Can you work these out from the model? Positions are in its coordinate system, mm. Round coordinates to 2 decimals unless told otherwise and drop trailing zeros. Order: outer loops, then holes, each group sorted by start corner. A loop starts at its lowest first (then second) coordinate and runs counter-clockwise, first axis right, second up. Notation, with made-up numbers: M 20,10.5 L 66,10.5 A16 ccw 66,39.5 Z; hole C -29,63 d11. An arc over 180 degrees is marked long. One line per question, with ' | ' between items.
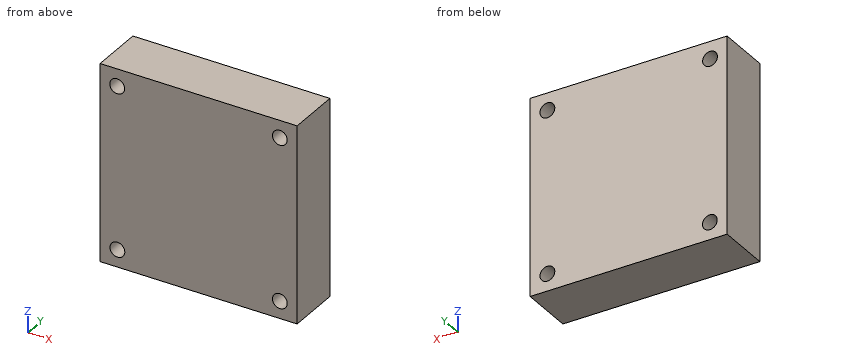
Autodesk Inventor part; units mm, degrees
ref_plane "YZ Plane" through (0, 0, 0) normal (1, 0, 0) x (0, 1, 0)
ref_plane "XZ Plane" through (0, 0, 0) normal (0, 1, 0) x (-1, 0, 0)
ref_plane "XY Plane" through (0, 0, 0) normal (0, 0, 1) x (1, 0, 0)
sketch "Sketch1" plane through (0, 0, 0) normal (0, 1, 0) x (-1, 0, 0)
  line L0 (-22.0009, 16.7182) -> (-22.0009, -23.1818)
  line L1 (-22.0009, -23.1818) -> (17.8991, -23.1818)
  line L2 (17.8991, -23.1818) -> (17.8991, 16.7182)
  line L3 (17.8991, 16.7182) -> (-22.0009, 16.7182)
  circle A0 centre (14.3991, -19.6818) radius 1.5
  circle A1 centre (14.4378, 13.2182) radius 1.5
  circle A2 centre (-18.5009, 13.2182) radius 1.5
  circle A3 centre (-18.5009, -19.6818) radius 1.5
  point P0 (0, 0)
  dimension "d0" = 39.9
  dimension "d2" = 39.9
  dimension "d3" = 3
  dimension "d4" = 3
  dimension "d5" = 3
  dimension "d6" = 3
  dimension "d7" = 3.5
  dimension "d8" = 3.5
  dimension "d9" = 3.5
  dimension "d10" = 3.5
  dimension "d11" = 3.5
  dimension "d12" = 3.5
  dimension "d13" = 3.5
extrude "Extrusion1" add sketch "Sketch1" along normal blind 10.8
properties part number "ventilator"
(1) If we section it at A-A on z = 12.5: Please give me the cut outline in (x, y), plus the area to 3 significant figures.
Final values:
outline: M -17.9,0 L -15.75,0 L -15.75,10.8 L -17.9,10.8 Z; M -13.12,0 L 17.18,0 L 17.18,10.8 L -13.12,10.8 Z; M 19.82,0 L 22,0 L 22,10.8 L 19.82,10.8 Z | area: 374 mm^2
(2) Please list where these lines run through material, in increasing order: probe 1 along X at (y, z) = (9.5, -19.5); probe 2 along X at (y, z) = (0.5, -20.5); probe 3 along Z at (x, y) = (-14, 2.25). Write a range as [from, to].
Final values:
probe 1: [-17.9, -15.89], [-12.91, 17.01], [19.99, 22] | probe 2: [-17.9, -15.66], [-13.14, 17.24], [19.76, 22] | probe 3: [-23.18, -21.13], [-18.24, 11.78], [14.65, 16.72]
(3) Will this pin go through, and if not, where does the flat tip stop? pin 1 Ø2.5 at (x, z) = (18.5, -19.68) entering from -Y.
Final values:
pin 1: through
(4) If we section it at B-B on y = 8.25: Please give me the cut outline in (x, z), plus the area to 3 significant figures.
Final values:
outline: M -17.9,-23.18 L 22,-23.18 L 22,16.72 L -17.9,16.72 Z; hole C -14.44,13.22 d3; hole C -14.4,-19.68 d3; hole C 18.5,-19.68 d3; hole C 18.5,13.22 d3 | area: 1,560 mm^2
(5) If we section it at C-C on x = 19.5: Please give me the cut outline in (y, z).
Final values:
outline: M 0,-23.18 L 10.8,-23.18 L 10.8,-20.8 L 0,-20.8 Z; M 0,-18.56 L 10.8,-18.56 L 10.8,12.1 L 0,12.1 Z; M 0,14.34 L 10.8,14.34 L 10.8,16.72 L 0,16.72 Z
